from build123d import *

# Parameters (mm, degrees)
SKETCH_1_R          = 3.5
EXTRUDE_1_DEPTH     = 3.91
SKETCH_2_R          = 2
EXTRUDE_2_DEPTH     = 70
CUT_EXTRUDE_1_DEPTH = 2
CHAMFER_1_SIZE      = 0.4
CHAMFER_2_SIZE      = 0.3


with BuildPart() as part:
    # 草图1 → 凸台-拉伸1 (new body)
    with BuildSketch(Plane.XY):
        Circle(SKETCH_1_R)
    extrude(amount=EXTRUDE_1_DEPTH)

    # 草图2 → 凸台-拉伸2 (add)
    with BuildSketch(Plane.XY.offset(3.91)):
        Circle(SKETCH_2_R)
    extrude(amount=EXTRUDE_2_DEPTH)

    # 草图3 → 切除-拉伸1 (cut)
    with BuildSketch(Plane(origin=(0, 0, 0), x_dir=(-1, 0, 0), z_dir=(0, 0, -1))):
        Polygon((0, 1.760918321), (-1.525, 0.880459161), (-1.525, -0.880459161), (0, -1.760918321), (1.525, -0.880459161), (1.525, 0.880459161), align=None)
    extrude(amount=-CUT_EXTRUDE_1_DEPTH, mode=Mode.SUBTRACT)

    # 倒角1
    chamfer_1_edges = [part.edges().sort_by_distance(p)[0] for p in [
        (-2, 0, 73.91),
    ]]
    chamfer(chamfer_1_edges, length=CHAMFER_1_SIZE)

    # 倒角2
    chamfer_2_edges = [part.edges().sort_by_distance(p)[0] for p in [
        (-3.5, 0, 0),
        (-3.5, 0, 3.91),
    ]]
    chamfer(chamfer_2_edges, length=CHAMFER_2_SIZE)


solid = part.part
Input: part model. Units: mm. Frame: model coordinates. A direction names the side the tool comes from. Coordinates: 2 decimals unless noted, no trailing zeros. Loops run counter-clockwise (first coordinate to the right, second up) from the corner with the lowest first, then second, coordinate; pieces in that order, holes last. Notation, with made-up numbers: (75, 18.25) -> (130, 18.25) arc R20 cw to (130, 33.25) -> close; hole circle Ø11 at (-12.5, 45.25). An arc over 180 degrees is marked (long way). Write item = value, one per line. Start each with the question number.
Item 1: Cut plane A-A, the plane y = 0. Return loops of the section in (x, z) (3 decimals).
Item 2: Material intervals for line 1 (Z direction, x = -0.25, y = 2.25); line 2 (Y direction, x = 0, z = 70); line 3 (Z direction, x = -1.25, y = -0.5), sorted ascending.
Item 3: Cut plane B-B, the plane z = 39. Return loops of the section in (x, y).
Item 4: First-contact query: P1, Ø4, axis at x = -2.5, z = 64.5, coming from the +Y side; P2, Ø0.5, axis at y = 0.5, z = 0.5, coming from the -X side; P3, Ø0.5, axis at y = 0.5, z = 0.5, coming from the +X side. Flat tips, straight axial feed; report the tip coordinate or a pass-through.
Item 5: Mould query, pull axis X, two halves, no side actions, for faces 1 (the face through (1.525, 0, 1)), 2 (the face through (0, 0, 73.91)), 3 (the face through (3.233, -1.341, 1.932)). Classes: pulls with the +X half, pulls with the -X half, needs draft (parallel to the pull), parting line crosses it, or undercut.
Item 6: Reachability of faces 4 (the face through (-0.8, 1.5, 0)), 5 (the face through (0, -2, 38)), 6 (the face through (-0.8, -1.3, 1)) from +Z, -Z, +X, -X, +Y, -Y: full face, straight path, thin tool, end or side. Return the list, or none.
Ans:
q1.outline = (-3.5, 0.3) -> (-3.2, 0) -> (-1.525, 0) -> (-1.525, 2) -> (1.525, 2) -> (1.525, 0) -> (3.2, 0) -> (3.5, 0.3) -> (3.5, 3.61) -> (3.2, 3.91) -> (2, 3.91) -> (2, 73.51) -> (1.6, 73.91) -> (-1.6, 73.91) -> (-2, 73.51) -> (-2, 3.91) -> (-3.2, 3.91) -> (-3.5, 3.61) -> close
q2.line_1 = 0 to 3.91
q2.line_2 = -2 to 2
q2.line_3 = 2 to 73.91
q3.outline = circle Ø4 at (0, 0)
q4.P1 = 1.94
q4.P2 = -3.49
q4.P3 = 3.49
q5.face_1 = undercut
q5.face_2 = needs draft
q5.face_3 = parting line crosses it
q6.face_4 = -Z, +X, -X, +Y, -Y
q6.face_5 = +Z
q6.face_6 = -Z
